from build123d import *

# Parameters (mm, degrees)
BOSS_EXTRUDE1_DEPTH = 25.4
SKETCH2_R           = 2.25
CUT_EXTRUDE1_DEPTH  = 44.249277532
SKETCH3_R           = 5.5
BOSS_EXTRUDE2_DEPTH = 4.7625
FILLET1_R           = 4


with BuildPart() as part:
    # Sketch1 → Boss-Extrude1 (new body)
    with BuildSketch(Plane(origin=(0, 0, 0), x_dir=(1, 0, 0), z_dir=(0, 1, 0))):
        Polygon((-6.5, 18.750739811), (-1.5, 21.642901866), (-1.5, 32.503507515), (-6.5, 32.503507515), align=None)
        with BuildLine():
            Line((-1.5, -21.625070485), (-1.5, -14.221111068))
            ThreePointArc((-1.5, -14.221111068), (-14.3, 0), (-1.5, 14.221111068))
            Line((-1.5, 14.221111068), (-1.5, 21.642901866))
            Line((-1.5, 21.642901866), (-6.5, 18.750739811))
            Line((-6.5, 18.750739811), (-19.494691465, 11.234189098))
            Line((-19.494691465, 11.234189098), (-19.476438882, -11.265803499))
            Line((-19.476438882, -11.265803499), (-6.5, -18.743724782))
            Line((-6.5, -18.743724782), (-1.5, -21.625070485))
        make_face()
        Polygon((-1.5, -32.496492485), (-1.5, -21.625070485), (-6.5, -18.743724782), (-6.5, -32.496492485), align=None)
    extrude(amount=BOSS_EXTRUDE1_DEPTH)

    # Sketch2 → Cut-Extrude1 (cut, through all)
    with BuildSketch(Plane.ZY.offset(6.5)):
        with Locations((25.620108634, 18.7)):
            Circle(SKETCH2_R)
        with Locations((25.620108634, 6.7)):
            Circle(SKETCH2_R)
    cut_extrude1 = extrude(amount=-CUT_EXTRUDE1_DEPTH, mode=Mode.SUBTRACT)

    # Mirror1: Cut-Extrude1 across plane
    add(cut_extrude1.mirror(Plane.XY), mode=Mode.SUBTRACT)

    # Sketch3 → Boss-Extrude2 (add)
    with BuildSketch(Plane(origin=(0, 25.4, 0), x_dir=(1, 0, 0), z_dir=(0, 1, 0))):
        Polygon((-100, 9.984192799), (-100, -10.015807201), (-19.476438882, -11.265803499), (-19.494691465, 11.234189098), align=None)
        with Locations(Location((-60, -0.015807201, 0), (0, 0, 270))):
            Circle(SKETCH3_R, mode=Mode.SUBTRACT)
        with Locations(Location((-75, -0.015807201, 0), (0, 0, 270))):
            Circle(SKETCH3_R, mode=Mode.SUBTRACT)
        with Locations(Location((-90, -0.015807201, 0), (0, 0, 270))):
            Circle(SKETCH3_R, mode=Mode.SUBTRACT)
    extrude(amount=-BOSS_EXTRUDE2_DEPTH)

    # Fillet1
    fillet1_edges = [part.edges().sort_by_distance(p)[0] for p in [
        (-100, 23.01875, 10.015807201),
        (-100, 23.01875, -9.984192799),
    ]]
    fillet(fillet1_edges, radius=FILLET1_R)


solid = part.part
For this review, take the finished solid that the model builds, in its own axes (mm). A direction names the side the tool comes from. Give positions to 0.01 mm unless a question says otherwise; leave off trailing zeros. Loops run counter-clockwise (first coordinate to the right, second up) from the corner with the lowest first, then second, coordinate; pieces in that order, holes last.
Item 1: Take a section at D-D, the plane z = 25. State the section outline as (x, y) points, and give its area (3 significant figures).
Item 2: Draft analysis for pull direction X (two halves, no side actions). For faces 4 (the cylindrical face through (-69.547, 23.052, -0.7)), 5 (the flat face through (-4, 13, -32.504)), 6 (the cylindrical face through (-84.547, 23.052, -0.7)), 7 (the flat face through (-1.5, 13, 23)), state which applies: +X half, -X half, draft (parallel to the pull), parting line (faces both ways), or undercut.
Item 3: For line 1 along X through (y, z) = (12.25, -25.5); line 2 along Z through (x, y) = (-85, 23); line 3 along X through (y, z) = (7.25, -18.5), list the stretches that pass through material, from the lowest coordinate up.
Item 4: Take a section at A-A, the plane y = 6.7. State the section outline as (x, z) points.
Item 5: Tool access review of faces 1 (the flat face through (-6.5, 13, -26)), 2 (the flat face through (-6.5, 13, 26)), 3 (the flat face through (-51, 20.638, 0)): name each direction out of +Z, -Z, +X, -X, +Y, -Y from which nothing blocks a thin tool from reaching the whole face with its end or side.
Item 6: Insertion check: pin 1 (11 mm diameter, centred on y = 18.5, z = -24, fed in from -X); pin 2 (12.5 mm diameter, centred on x = -75, z = 0.02, fed in from +Y); pin 3 (12 mm diameter, centred on y = 4, z = 11.5, fed in from -X); pin 4 (4 mm diameter, centred on x = -19.5, y = 20, fed in from +Z). Each pin has a flat end and moves straight along its axis. Give the tip position at first contact, or say it passes through.
Item 7: Take a section at B-B, the plane x = -90. State the section outline as (y, z) points, and give its area (3 significant figures).
Item 8: Take a section at C-C, the plane z = 3. State the section outline as (x, y) points.
Calculated:
1. outline: (-6.5, 0) - (-1.5, 0) - (-1.5, 4.54) - (-6.5, 4.54) - close; (-6.5, 8.86) - (-1.5, 8.86) - (-1.5, 16.54) - (-6.5, 16.54) - close; (-6.5, 20.86) - (-1.5, 20.86) - (-1.5, 25.4) - (-6.5, 25.4) - close
1. area: 83.7 mm2
2. face 4: undercut
2. face 5: draft
2. face 6: undercut
2. face 7: +X half
3. line 1: x = -6.5 to -1.5
3. line 2: z = -10.22 to -2.28, 2.31 to 10.25
3. line 3: x = -6.93 to -1.5
4. outline: (-19.49, -11.23) - (-6.5, -18.75) - (-6.5, -23.37) - (-1.5, -23.37) - (-1.5, -14.22) arc R14.3 cw to (-1.5, 14.22) - (-1.5, 23.37) - (-6.5, 23.37) - (-6.5, 18.74) - (-19.48, 11.27) - close; (-6.5, -32.5) - (-1.5, -32.5) - (-1.5, -27.87) - (-6.5, -27.87) - close; (-6.5, 27.87) - (-1.5, 27.87) - (-1.5, 32.5) - (-6.5, 32.5) - close
5. face 1: -Z, -X, +Y, -Y
5. face 2: +Z, -X, +Y, -Y
5. face 3: +Z, -Z, -X, -Y
6. pin 1: stops at x = -6.93
6. pin 2: stops at y = 25.4
6. pin 3: stops at x = -19.48
6. pin 4: stops at z = 12.4
7. outline: (20.64, -10.14) - (25.4, -10.14) - (25.4, -5.48) - (20.64, -5.48) - close; (20.64, 5.52) - (25.4, 5.52) - (25.4, 10.17) - (20.64, 10.17) - close
7. area: 44.3 mm2
8. outline: (-100, 20.64) - (-94.62, 20.64) - (-94.62, 25.4) - (-100, 25.4) - close; (-85.38, 20.64) - (-79.62, 20.64) - (-79.62, 25.4) - (-85.38, 25.4) - close; (-70.38, 20.64) - (-64.62, 20.64) - (-64.62, 25.4) - (-70.38, 25.4) - close; (-55.38, 20.64) - (-19.48, 20.64) - (-19.48, 0) - (-13.98, 0) - (-13.98, 25.4) - (-55.38, 25.4) - close
